from build123d import *

# Parameters (mm, degrees)
CUT_EXTRUDE1_REACH = 18.111


with BuildPart() as part:
    # Sketch1 → Revolve1 (revolve)
    with BuildSketch(Plane.XY, mode=Mode.PRIVATE) as revolve1_sk:
        Polygon((-4.75, 0), (-4.75, 6.8), (-6.6, 6.8), (-6.6, 16.7), (-4, 16.7), (-4, 17.7), (-6.825, 17.7), (-6.825, 19.7), (-3, 19.7), (-3, 0), align=None)
    revolve(revolve1_sk.sketch.rotate(Axis((0, 0, 0), (0, 1, 0)), 270), axis=Axis((0, 0, 0), (0, 1, 0)))

    # Sketch2 → Cut-Extrude1 (cut, up to next)
    with BuildSketch(Plane.XZ.offset(-6.8), mode=Mode.PRIVATE) as cut_extrude1_sk1:
        with BuildLine():
            Line((-5.715767665, 3.3), (0, 6.6))
            ThreePointArc((0, 6.6), (-3.3, 5.715767665), (-5.715767665, 3.3))
        make_face()
    cut_extrude1_tool1 = extrude(cut_extrude1_sk1.sketch, amount=-CUT_EXTRUDE1_REACH, mode=Mode.PRIVATE) & part.part
    # Sketch2 → Cut-Extrude1 (cut, up to next)
    with BuildSketch(Plane.XZ.offset(-6.8), mode=Mode.PRIVATE) as cut_extrude1_sk2:
        with BuildLine():
            ThreePointArc((5.715767665, 3.3), (3.3, 5.715767665), (0, 6.6))
            Line((0, 6.6), (5.715767665, 3.3))
        make_face()
    cut_extrude1_tool2 = extrude(cut_extrude1_sk2.sketch, amount=-CUT_EXTRUDE1_REACH, mode=Mode.PRIVATE) & part.part
    # Sketch2 → Cut-Extrude1 (cut, up to next)
    with BuildSketch(Plane.XZ.offset(-6.8), mode=Mode.PRIVATE) as cut_extrude1_sk3:
        with BuildLine():
            ThreePointArc((6.6, 0), (6.375110454, 1.708205698), (5.715767665, 3.3))
            Line((5.715767665, 3.3), (5.715767665, -3.3))
            ThreePointArc((5.715767665, -3.3), (6.375110454, -1.708205698), (6.6, 0))
        make_face()
    cut_extrude1_tool3 = extrude(cut_extrude1_sk3.sketch, amount=-CUT_EXTRUDE1_REACH, mode=Mode.PRIVATE) & part.part
    # Sketch2 → Cut-Extrude1 (cut, up to next)
    with BuildSketch(Plane.XZ.offset(-6.8), mode=Mode.PRIVATE) as cut_extrude1_sk4:
        with BuildLine():
            ThreePointArc((0, -6.6), (3.3, -5.715767665), (5.715767665, -3.3))
            Line((5.715767665, -3.3), (0, -6.6))
        make_face()
    cut_extrude1_tool4 = extrude(cut_extrude1_sk4.sketch, amount=-CUT_EXTRUDE1_REACH, mode=Mode.PRIVATE) & part.part
    # Sketch2 → Cut-Extrude1 (cut, up to next)
    with BuildSketch(Plane.XZ.offset(-6.8), mode=Mode.PRIVATE) as cut_extrude1_sk5:
        with BuildLine():
            Line((0, -6.6), (-5.715767665, -3.3))
            ThreePointArc((-5.715767665, -3.3), (-3.3, -5.715767665), (0, -6.6))
        make_face()
    cut_extrude1_tool5 = extrude(cut_extrude1_sk5.sketch, amount=-CUT_EXTRUDE1_REACH, mode=Mode.PRIVATE) & part.part
    # Sketch2 → Cut-Extrude1 (cut, up to next)
    with BuildSketch(Plane.XZ.offset(-6.8), mode=Mode.PRIVATE) as cut_extrude1_sk6:
        with BuildLine():
            Line((-5.715767665, -3.3), (-5.715767665, 3.3))
            ThreePointArc((-5.715767665, 3.3), (-6.6, 0), (-5.715767665, -3.3))
        make_face()
    cut_extrude1_tool6 = extrude(cut_extrude1_sk6.sketch, amount=-CUT_EXTRUDE1_REACH, mode=Mode.PRIVATE) & part.part
    add(cut_extrude1_tool1.solids().sort_by_distance((-3.035787, 6.8, 5.258137))[0], mode=Mode.SUBTRACT)
    add(cut_extrude1_tool2.solids().sort_by_distance((3.035787, 6.8, 5.258137))[0], mode=Mode.SUBTRACT)
    add(cut_extrude1_tool3.solids().sort_by_distance((6.071573, 6.8, 0))[0], mode=Mode.SUBTRACT)
    add(cut_extrude1_tool4.solids().sort_by_distance((3.035787, 6.8, -5.258137))[0], mode=Mode.SUBTRACT)
    add(cut_extrude1_tool5.solids().sort_by_distance((-3.035787, 6.8, -5.258137))[0], mode=Mode.SUBTRACT)
    add(cut_extrude1_tool6.solids().sort_by_distance((-6.071573, 6.8, 0))[0], mode=Mode.SUBTRACT)


solid = part.part
Verification items for the finished model (mm, model axes). A direction names the side the tool comes from. Coordinates: 2 decimals unless noted, no trailing zeros. Order: outer loops, then holes, each group sorted by start corner. A loop starts at its lowest first (then second) coordinate and runs counter-clockwise, first axis right, second up.
Item 1: Depth check by flat-ended pin: pin 1 (6 mm diameter, centred on y = 5.5, z = -2, fed in from +X); pin 2 (1.5 mm diameter, centred on x = -2.5, y = 10.5, fed in from -Z); pin 3 (2 mm diameter, centred on y = 5.5, z = -1.5, fed in from +X). Enter the tip coordinate at first touch or a pass-through.
Filled in:
pin 1: stops at x = 5.72
pin 2: stops at z = -5.59
pin 3: stops at x = 4.72
Item 2: Section check B-B, the plane y = 11.75. Enter the section's corners in (x, z).
Filled in:
outline: (-5.72, -3.3) - (0, -6.6) - (5.72, -3.3) - (5.72, 3.3) - (0, 6.6) - (-5.72, 3.3) - close; hole circle Ø6 at (0, 0)
Item 3: Access from +Z, -Z, +X, -X, +Y, -Y to the whole of each face (thin tool, end or side, straight path). Record for faces 4 (the face through (2.82, 11.68, 4.97)), 5 (the face through (3, 17.7, 3)), 6 (the face through (-2.898, 11.681, 4.927)), 7 (the face through (-5.716, 12, 0)).
Filled in:
face 4: +Z, +X, -Y
face 5: none
face 6: +Z, -X, -Y
face 7: +Z, -Z, -X, -Y
Item 4: Release check for a two-part mould opening along Z. For faces 1 (the face through (1, 19.7, -3)), 2 (the face through (2.89, 3.45, 3.77)), 3 (the face through (-0.9, 9.71, -2.86)) record: +Z half, -Z half, draft (parallel to the pull), parting line (faces both ways), or undercut.
Filled in:
face 1: draft
face 2: parting line
face 3: undercut
Item 5: Section check C-C, the plane x = 0.5. Enter the section's corners in (y, z), then the cut area to 3 significant figures.
Filled in:
outline: (0, -4.72) - (6.8, -4.72) - (6.8, -6.31) - (16.7, -6.31) - (16.7, -3.97) - (17.7, -3.97) - (17.7, -6.81) - (19.7, -6.81) - (19.7, -2.96) - (0, -2.96) - close; (0, 2.96) - (19.7, 2.96) - (19.7, 6.81) - (17.7, 6.81) - (17.7, 3.97) - (16.7, 3.97) - (16.7, 6.31) - (6.8, 6.31) - (6.8, 4.72) - (0, 4.72) - close
area: 108 mm2
Item 6: Material ranges on L1, parallel to X at y = 13.5, z = 0; L2, parallel to X at y = 4, z = 0; L3, parallel to Y at x = -4.75, z = 1, recorded low to high.
Filled in:
L1: x = -5.72 to -3, 3 to 5.72
L2: x = -4.75 to -3, 3 to 4.75
L3: y = 6.8 to 16.7, 17.7 to 19.7
Item 7: Section check A-A, the plane z = 0. Enter the section's corners in (x, y) (3 decimals).
Filled in:
outline: (-6.825, 17.7) - (-4, 17.7) - (-4, 16.7) - (-5.716, 16.7) - (-5.716, 6.8) - (-4.75, 6.8) - (-4.75, 0) - (-3, 0) - (-3, 19.7) - (-6.825, 19.7) - close; (3, 0) - (4.75, 0) - (4.75, 6.8) - (5.716, 6.8) - (5.716, 16.7) - (4, 16.7) - (4, 17.7) - (6.825, 17.7) - (6.825, 19.7) - (3, 19.7) - close
Item 8: Section check D-D, the plane z = -4.25. Enter the section's corners in (x, y), then the cut area to 3 significant figures.
Filled in:
outline: (-5.34, 17.7) - (5.34, 17.7) - (5.34, 19.7) - (-5.34, 19.7) - close; (-4.07, 6.8) - (-2.12, 6.8) - (-2.12, 0) - (2.12, 0) - (2.12, 6.8) - (4.07, 6.8) - (4.07, 16.7) - (-4.07, 16.7) - close
area: 131 mm2
